For this review, take the finished solid that the model builds, in its own axes (mm). A direction names the side the tool comes from. Give positions to 0.01 mm unless a question says otherwise; leave off trailing zeros. Loops run counter-clockwise (first coordinate to the right, second up) from the corner with the lowest first, then second, coordinate; pieces in that order, holes last. Notation, with made-up numbers: (77, -39) - (114, -39) arc R32 cw to (114, -11) - close; hole circle Ø8 at (-32.5, 4). An arc over 180 degrees is marked (long way). Use CSV: the item, a comma, the result in double quotes. Start each with the question number.
1. Mouldability with a two-part tool opening along X and no side actions: class faces 1 (the flat face through (2, 0, 1)), 2 (the cylindrical face through (-3.25, -2.21, 4.23)), 3 (the cylindrical face through (1.93, 4.83, 2.52)), 4 (the flat face through (4, -52.388, -1)) as pulls with the +X half, pulls with the -X half, needs draft (parallel to the pull), parting line crosses it, or undercut.
2. For faces 5 (the flat face through (4, -14.288, -1)), 6 (the flat face through (3.5, 9.525, -0.1)), list the 3-axis set-ups (+Z, -Z, +X, -X, +Y, -Y) from which the entire face can be reached by the end or side of a thin tool; tool diameter is ignored.
3. Take a section at C-C on y = -59. Give the boundary of the cut face in (x, z), plus the area to 3 significant figures.
4. Take a section at D-D on y = -18. Give the boundary of the cut face in (x, z), plus the area to 3 significant figures.
5. Take a section at A-A on x = 0. Give the boundary of the cut face in (y, z) (1 decimal).
6. For pin 1 (1.5 mm diameter, centred on x = -1.5, y = -54.5, fed in from +Z); pin 2 (1 mm diameter, centred on x = 2, y = -33, fed in from +Z); pin 3 (1 mm diameter, centred on y = -40.5, z = 1.5, fed in from -X), all flat-tipped, find the tip position at first contact; note any pin that passes through.
7. Take a section at B-B on z = 0. Give the boundary of the cut face in (x, y) (1 decimal), plus the area to 3 significant figures.
8. Wall thickness on line 1 (Y direction, x = 1.75, z = 4.5) (1 decimal); line 2 (X direction, y = -4, z = 0): over which ranges is each line inside the solid? List them lowest first.
```python
from build123d import *

# Parameters (mm, degrees)
SKETCH2_R           = 5.334
SKETCH2_R_2         = 2
BOSS_EXTRUDE1_DEPTH = 61.9125
CUT_EXTRUDE1_START  = -19.05
SKETCH3_R           = 5.334
SKETCH3_R_2         = 3.7465
CUT_EXTRUDE1_DEPTH  = 38.1


with BuildPart() as part:
    # Sketch1 → Revolve1 (revolve)
    with BuildSketch(Plane.XY, mode=Mode.PRIVATE) as revolve1_sk:
        Polygon((2, 0), (3.175, 0), (3.175, 9.525), (5.334, 9.525), (5.334, -9.525), (2, -9.525), align=None)
    revolve(revolve1_sk.sketch.rotate(Axis((0, 0, 0), (0, 1, 0)), 90), axis=Axis((0, 0, 0), (0, 1, 0)))

    # Sketch2 → Boss-Extrude1 (add)
    with BuildSketch(Plane.XZ.offset(9.525)):
        with Locations(Location((0, 0, 0), (0, 0, 270))):
            Circle(SKETCH2_R)
        with Locations(Location((0, 0, 0), (0, 0, 270))):
            Circle(SKETCH2_R_2, mode=Mode.SUBTRACT)
    extrude(amount=BOSS_EXTRUDE1_DEPTH)

    # Sketch3 → Cut-Extrude1 (cut)
    with BuildSketch(Plane.XZ.offset(71.4375).offset(CUT_EXTRUDE1_START)):
        with Locations(Location((0, 0, 0), (0, 0, 270))):
            Circle(SKETCH3_R)
        with Locations(Location((0, 0, 0), (0, 0, 270))):
            Circle(SKETCH3_R_2, mode=Mode.SUBTRACT)
    extrude(amount=-CUT_EXTRUDE1_DEPTH, mode=Mode.SUBTRACT)


solid = part.part
```
Check result:
1,face 1,"undercut"
1,face 2,"parting line crosses it"
1,face 3,"undercut"
1,face 4,"needs draft"
2,face 5,"none"
2,face 6,"+Z, -Z, +X, -X, +Y"
3,outline,"circle Ø10.67 at (0, 0); hole circle Ø4 at (0, 0)"
3,area,"76.8 mm²"
4,outline,"circle Ø7.49 at (0, 0); hole circle Ø4 at (0, 0)"
4,area,"31.5 mm²"
5,outline,"(-71.4, -5.3) - (-52.4, -5.3) - (-52.4, -3.7) - (-14.3, -3.7) - (-14.3, -5.3) - (9.5, -5.3) - (9.5, -3.2) - (0, -3.2) - (0, -2) - (-71.4, -2) - close; (-71.4, 2) - (0, 2) - (0, 3.2) - (9.5, 3.2) - (9.5, 5.3) - (-14.3, 5.3) - (-14.3, 3.7) - (-52.4, 3.7) - (-52.4, 5.3) - (-71.4, 5.3) - close"
6,pin 1,"stops at z = 5.28"
6,pin 2,"stops at z = 3.43"
6,pin 3,"stops at x = -3.61"
7,outline,"(-5.3, -71.4) - (-2, -71.4) - (-2, 0) - (-3.2, 0) - (-3.2, 9.5) - (-5.3, 9.5) - (-5.3, -14.3) - (-3.7, -14.3) - (-3.7, -52.4) - (-5.3, -52.4) - close; (2, -71.4) - (5.3, -71.4) - (5.3, -52.4) - (3.7, -52.4) - (3.7, -14.3) - (5.3, -14.3) - (5.3, 9.5) - (3.2, 9.5) - (3.2, 0) - (2, 0) - close"
7,area,"397 mm²"
8,line 1,"y = -71.4 to -52.4, -14.3 to 9.5"
8,line 2,"x = -5.33 to -2, 2 to 5.33"
